from build123d import *

# Parameters (mm, degrees)
SKETCH_1_R          = 10
EXTRUDE_1_DEPTH     = 1
SKETCH_2_R          = 4.5
EXTRUDE_2_DEPTH     = 0.5
CHAMFER_1_SIZE      = 0.5
SKETCH_3_R          = 1.75
CUT_EXTRUDE_1_DEPTH = 15.221462653
SKETCH_4_R          = 0.5
CUT_EXTRUDE_2_DEPTH = 15.221462653


with BuildPart() as part:
    # 草图1 → 凸台-拉伸1 (new body)
    with BuildSketch(Plane.XY):
        Circle(SKETCH_1_R)
    extrude(amount=EXTRUDE_1_DEPTH)

    # 草图2 → 凸台-拉伸2 (add)
    with BuildSketch(Plane.XY.offset(1)):
        Circle(SKETCH_2_R)
    extrude(amount=EXTRUDE_2_DEPTH)

    # 倒角1
    chamfer_1_edges = [part.edges().sort_by_distance(p)[0] for p in [
        (-4.5, 0, 1.5),
    ]]
    chamfer(chamfer_1_edges, length=CHAMFER_1_SIZE - 0.0001)  # a hair under: the kernel refuses the full size

    # 草图3 → 切除-拉伸1 (cut, through all)
    with BuildSketch(Plane(origin=(0, 0, 0), x_dir=(-1, 0, 0), z_dir=(0, 0, -1))):
        Circle(SKETCH_3_R)
    extrude(amount=-CUT_EXTRUDE_1_DEPTH, mode=Mode.SUBTRACT)

    # 草图4 → 切除-拉伸2 (cut, through all)
    with BuildSketch(Plane(origin=(0, 0, 0), x_dir=(-1, 0, 0), z_dir=(0, 0, -1))):
        with Locations((0, 8)):
            Circle(SKETCH_4_R)
        with Locations((8, 0)):
            Circle(SKETCH_4_R)
        with Locations((0, -8)):
            Circle(SKETCH_4_R)
        with Locations((-8, 0)):
            Circle(SKETCH_4_R)
    extrude(amount=-CUT_EXTRUDE_2_DEPTH, mode=Mode.SUBTRACT)


solid = part.part
Geometry check sheet. Reference: the model listing, model coordinates, mm. A direction names the side the tool comes from. Give positions to 0.01 mm unless a question says otherwise; leave off trailing zeros. Loops run counter-clockwise (first coordinate to the right, second up) from the corner with the lowest first, then second, coordinate; pieces in that order, holes last. Notation, with made-up numbers: M 42,28.25 L 89,28.25 A17 ccw 89,53.25 Z; hole C 86.25,70 d2. An arc over 180 degrees is marked long. Answer as a JSON object with one key per item and string values. Group by question number.
Item 1: Material ranges on L1, parallel to Y at x = -0.25, z = 0.4; L2, parallel to Z at x = -6, y = -7.5; L3, parallel to Y at x = 2.75, z = 1.35, recorded low to high.
Item 2: Sectioned sample at B-B on y = -8. Record the boundary of the cut face in (x, z).
Item 3: Gauge pin test, flat end, axial feed: pin 1 (8 mm diameter, centred on x = 0.5, y = -1.5, fed in from +Z). Record the tip position at first contact, or that the pin passes through.
Item 4: Mould release check, pull along X, two halves, no side actions. Record for faces 3 (the cylindrical face through (-1.617, -0.67, 0.74)), 4 (the cylindrical face through (-2.17, -9.76, 0.49)), 5 (the flat face through (2, 0, 0)): pulls with the +X half, pulls with the -X half, needs draft (parallel to the pull), parting line crosses it, or undercut.
Item 5: Access from +Z, -Z, +X, -X, +Y, -Y to the whole of each face (thin tool, end or side, straight path). Record for faces 1 (the cylindrical face through (0.108, 7.512, 0.493)), 2 (the flat face through (4.3, -2.1, 1)).
Item 6: Sectioned sample at A-A on x = 0. Give the number of separate pieces and of enclosed holes in the cut face, plus the area to 3 significant figures.
Findings below:
{
 "1": {"L1": "-10 to -8.43, -7.57 to -1.73, 1.73 to 7.57, 8.43 to 10", "L2": "0 to 1", "L3": "-3.11 to 3.11"},
 "2": {"outline": "M -6,0 L -0.5,0 L -0.5,1 L -6,1 Z; M 0.5,0 L 6,0 L 6,1 L 0.5,1 Z"},
 "3": {"pin 1": "z = 1.5"},
 "4": {"face 3": "undercut", "face 4": "parting line crosses it", "face 5": "needs draft"},
 "5": {"face 1": "+Z, -Z", "face 2": "+Z"},
 "6": {"separate pieces": "4", "enclosed holes": "0", "area": "17.0 mm2"}
}
